Part print with two shaded views. Sizes in mm from the minimum x, y, z corner. A direction names the side the tool comes from. Coordinates: 2 decimals unless noted, no trailing zeros. Write each loop counter-clockwise with the first axis right and the second up, starting at its lowest first coordinate (ties: lowest second). Pieces come first, ordered by that corner, then holes.
Q1. Pin check, flat tips, straight feed: P1, Ø0.9, axis at x = 24.5, y = 13.5, coming from the +Z side; P2, Ø11, axis at y = 6.5, z = 23.5, coming from the -X side; P3, Ø1.8, axis at x = 28.5, z = 25.5, coming from the -Y side; P4, Ø12, axis at x = 10, z = 25, coming from the +Y side. Stop position of each tip, or through.
Q2. Which spindle directions (+Z, -Z, +X, -X, +Y, -Y) get a long thin tool onto all of the face, cutting with end or side? Do the marked faces 1, 2, 3, 4 and 5. Say none if no direction does.
Q3. Drill centre lines: probe 1 along Y at (x, z) = (91.5, 39.5); probe 2 along Z at (x, y) = (28.5, 4); probe 3 along X at (y, z) = (14, 26). Where is each one in solid material? Low to high.
Q4. Band-saw the part on D-D, the plane z = 45. Write the cut outline in (x, y).
Q5. Band-saw the part on A-A, the plane y = 14. Write the cut outline in (x, z), plus the area to 3 significant figures.
Q6. Band-saw the part on B-B, the plane x = 83.5. Write the cut outline in (y, z), plus the area to 3 significant figures.
Q7. Band-saw the part on C-C, the plane z = 15. Write the cut outline in (x, y), plus the area to 3 significant figures.
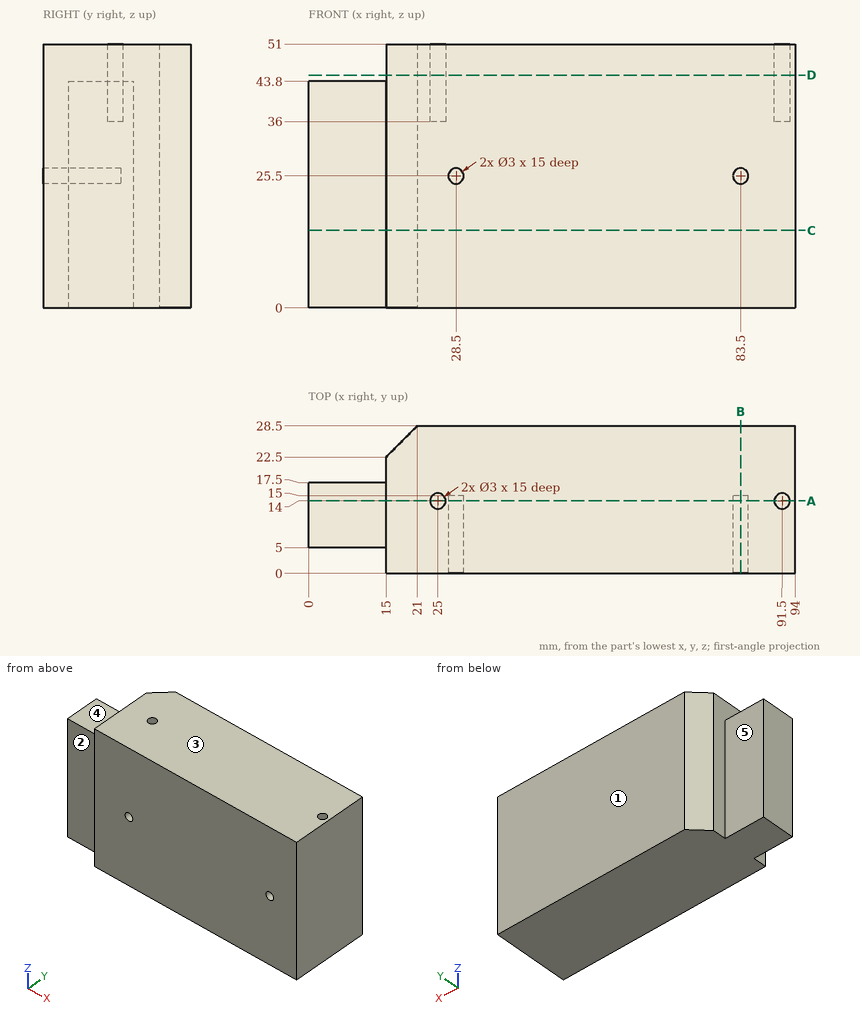
Answer sheet:
1. P1: stops at z = 36
1. P2: stops at x = 0
1. P3: stops at y = 15
1. P4: stops at y = 23.5
2. face 1: +Z, -Z, +X, -X, +Y
2. face 2: +Z, -Z, -X, -Y
2. face 3: +Z, +X, -X, +Y, -Y
2. face 4: +Z, -X, +Y, -Y
2. face 5: +Z, -Z, -X, +Y
3. probe 1: y = 0 to 12.5, 15.5 to 28.5
3. probe 2: z = 0 to 24, 27 to 51
3. probe 3: x = 0 to 27.09, 29.91 to 82.09, 84.91 to 94
4. outline: (15, 0) - (94, 0) - (94, 28.5) - (21, 28.5) - (15, 22.5) - close; hole circle Ø3 at (25, 14); hole circle Ø3 at (91.5, 14)
5. outline: (0, 0) - (94, 0) - (94, 51) - (93, 51) - (93, 36) - (90, 36) - (90, 51) - (26.5, 51) - (26.5, 36) - (23.5, 36) - (23.5, 51) - (15, 51) - (15, 43.8) - (0, 43.8) - close; hole circle Ø3 at (28.5, 25.5); hole circle Ø3 at (83.5, 25.5)
5. area: 4,580 mm2
6. outline: (0, 0) - (28.5, 0) - (28.5, 51) - (0, 51) - (0, 27) - (15, 27) - (15, 24) - (0, 24) - close
6. area: 1,410 mm2
7. outline: (0, 5) - (15, 5) - (15, 0) - (94, 0) - (94, 28.5) - (21, 28.5) - (15, 22.5) - (15, 17.5) - (0, 17.5) - close
7. area: 2,420 mm2
